```python
from build123d import *

# Parameters (mm, degrees)
SKETCH2_R           = 7.9375
BOSS_EXTRUDE1_DEPTH = 15.875
FILLET1_R           = 12.7
SKETCH3_R           = 22.225
CUT_EXTRUDE1_DEPTH  = 3.175
SKETCH4_R           = 4.7625
CUT_EXTRUDE2_DEPTH  = 6.35
SKETCH5_R           = 3.175
CUT_EXTRUDE3_DEPTH  = 115.871833471
SKETCH6_R           = 1.5875
CUT_EXTRUDE4_DEPTH  = 116.178567885
SKETCH7_W           = 66.04
SKETCH7_H           = 12.7
CUT_EXTRUDE5_DEPTH  = 116.571744492
FILLET2_R           = 3.175


with BuildPart() as part:
    # Sketch2 → Boss-Extrude1 (new body)
    # profile 1 of 5: a face of its own
    with BuildSketch(Plane(origin=(0, 0, 0), x_dir=(1, 0, 0), z_dir=(0, 1, 0))):
        with BuildLine():
            Line((-107.95, 0), (-107.95, -25.4))
            Line((-107.95, -25.4), (-21.997045256, -25.4))
            ThreePointArc((-21.997045256, -25.4), (-25.4, -12.7), (-21.997045256, 0))
            Line((-21.997045256, 0), (-107.95, 0))
        make_face()
    # profile 2 of 5: a face of its own
    with BuildSketch(Plane(origin=(0, 0, 0), x_dir=(1, 0, 0), z_dir=(0, 1, 0))):
        with BuildLine():
            ThreePointArc((-21.997045256, 0), (-25.4, -12.7), (-21.997045256, -25.4))
            Line((-21.997045256, -25.4), (-21.997045256, 0))
        make_face()
    # profile 3 of 5: a face of its own
    with BuildSketch(Plane(origin=(0, 0, 0), x_dir=(1, 0, 0), z_dir=(0, 1, 0))):
        with BuildLine():
            Line((-21.997045256, 0), (-21.997045256, -25.4))
            ThreePointArc((-21.997045256, -25.4), (0, -38.1), (21.997045256, -25.4))
            Line((21.997045256, -25.4), (21.997045256, 0))
            ThreePointArc((21.997045256, 0), (0, 12.7), (-21.997045256, 0))
        make_face()
        with Locations(Location((0, -12.7, 0), (0, 0, 270))):
            Circle(SKETCH2_R, mode=Mode.SUBTRACT)
    # profile 4 of 5: a face of its own
    with BuildSketch(Plane(origin=(0, 0, 0), x_dir=(1, 0, 0), z_dir=(0, 1, 0))):
        with BuildLine():
            Line((21.997045256, 0), (21.997045256, -25.4))
            ThreePointArc((21.997045256, -25.4), (24.534515988, -19.274003746), (25.4, -12.7))
            ThreePointArc((25.4, -12.7), (24.534515988, -6.125996254), (21.997045256, 0))
        make_face()
    # profile 5 of 5: a face of its own
    with BuildSketch(Plane(origin=(0, 0, 0), x_dir=(1, 0, 0), z_dir=(0, 1, 0))):
        with BuildLine():
            ThreePointArc((25.4, -12.7), (24.534515988, -19.274003746), (21.997045256, -25.4))
            Line((21.997045256, -25.4), (107.95, -25.4))
            Line((107.95, -25.4), (107.95, 0))
            Line((107.95, 0), (21.997045256, 0))
            ThreePointArc((21.997045256, 0), (24.534515988, -6.125996254), (25.4, -12.7))
        make_face()
    extrude(amount=BOSS_EXTRUDE1_DEPTH)

    # Fillet1
    fillet1_edges = [part.edges().sort_by_distance(p)[0] for p in [
        (-21.997045256, 7.9375, 0),
        (21.997045256, 7.9375, 0),
        (21.997045256, 7.9375, 25.4),
        (-21.997045256, 7.9375, 25.4),
    ]]
    fillet(fillet1_edges, radius=FILLET1_R)

    # Sketch3 → Cut-Extrude1 (cut)
    with BuildSketch(Plane.XZ):
        with Locations(Location((0, 12.7, 0), (0, 0, 270))):
            Circle(SKETCH3_R)
    extrude(amount=-CUT_EXTRUDE1_DEPTH, mode=Mode.SUBTRACT)

    # Sketch4 → Cut-Extrude2 (cut)
    with BuildSketch(Plane(origin=(0, 15.875, 0), x_dir=(1, 0, 0), z_dir=(0, 1, 0))):
        with Locations(Location((-101.6, -12.7, 0), (0, 0, 270))):
            Circle(SKETCH4_R)
        with Locations(Location((101.6, -12.7, 0), (0, 0, 270))):
            Circle(SKETCH4_R)
    extrude(amount=-CUT_EXTRUDE2_DEPTH, mode=Mode.SUBTRACT)

    # Sketch5 → Cut-Extrude3 (cut, through all)
    with BuildSketch(Plane(origin=(0, 9.525, 0), x_dir=(1, 0, 0), z_dir=(0, 1, 0))):
        with Locations(Location((-101.6, -12.7, 0), (0, 0, 270))):
            Circle(SKETCH5_R)
        with Locations(Location((101.6, -12.7, 0), (0, 0, 270))):
            Circle(SKETCH5_R)
    extrude(amount=-CUT_EXTRUDE3_DEPTH, mode=Mode.SUBTRACT)

    # Sketch6 → Cut-Extrude4 (cut, through all)
    with BuildSketch(Plane.XZ.offset(-3.175)):
        with Locations(Location((0, 29.21, 0), (0, 0, 270))):
            Circle(SKETCH6_R)
        with Locations(Location((14.298079416, 4.445, 0), (0, 0, 270))):
            Circle(SKETCH6_R)
        with Locations(Location((-14.298079416, 4.445, 0), (0, 0, 270))):
            Circle(SKETCH6_R)
    extrude(amount=-CUT_EXTRUDE4_DEPTH, mode=Mode.SUBTRACT)

    # Sketch7 → Cut-Extrude5 (cut, through all)
    with BuildSketch(Plane(origin=(0, 15.875, 0), x_dir=(1, 0, 0), z_dir=(0, 1, 0))):
        with Locations((-58.42, -12.7)):
            Rectangle(SKETCH7_W, SKETCH7_H)
        with Locations((58.42, -12.7)):
            Rectangle(SKETCH7_W, SKETCH7_H)
    extrude(amount=-CUT_EXTRUDE5_DEPTH, mode=Mode.SUBTRACT)

    # Fillet2
    fillet2_edges = [part.edges().sort_by_distance(p)[0] for p in [
        (-91.44, 7.9375, 19.05),
        (-91.44, 7.9375, 6.35),
        (-25.4, 7.9375, 6.35),
        (-25.4, 7.9375, 19.05),
        (25.4, 7.9375, 19.05),
        (25.4, 7.9375, 6.35),
        (91.44, 7.9375, 6.35),
        (91.44, 7.9375, 19.05),
    ]]
    fillet(fillet2_edges, radius=FILLET2_R)


solid = part.part
```
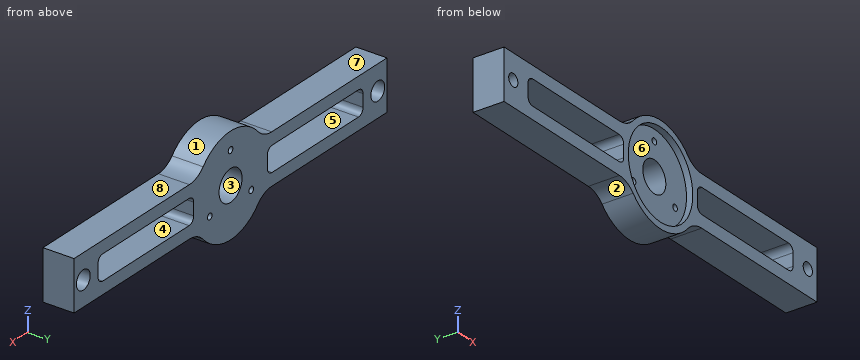
Build history of the part. All positions in model axes, mm. Face numbers are marked on the shaded views. A direction names the side the tool comes from. Round coordinates to 2 decimals unless told otherwise and drop trailing zeros. Loops run counter-clockwise (first coordinate to the right, second up) from the corner with the lowest first, then second, coordinate; pieces in that order, holes last. Notation, with made-up numbers: M 3,81.5 L 38,81.5 A8 cw 38,88.5 Z; hole C 47.5,12.25 d7. An arc over 180 degrees is marked long. Answer as CSV lines item,"result".
1. Flat gauge pins, fed straight in: P1, Ø8, axis at x = -2.5, z = 27.5, coming from the -Y side (3 decimals); P2, Ø1, axis at x = -9, y = 12, coming from the -Z side; P3, Ø5, axis at x = -65.5, y = 4, coming from the -Z side. Where does each tip first touch, or does it go through?
Resolved:
P1,"stops at y = 3.175"
P2,"stops at z = -11.24"
P3,"stops at z = 0"
2. Two-plate mould, pull along X, no slides. Class the marked faces 1, 2, 3 and 4: released by +X, released by -X, zero draft, split by the parting line, or undercut.
Resolved:
face 1,"split by the parting line"
face 2,"released by -X"
face 3,"undercut"
face 4,"undercut"
3. 3-axis set-ups, long thin cutter, end or side, ignore diameter. For the marked faces 5, 6, 7 and 8: which of +Z, -Z, +X, -X, +Y, -Y reach the whole face in a straight line?
Resolved:
face 5,"+Y, -Y"
face 6,"-Y"
face 7,"+Z, -X, +Y, -Y"
face 8,"+Z, +X, +Y, -Y"
4. Wall check: probe 1 along X at (y, z) = (11.25, 12.7); probe 2 along X at (y, z) = (11, 4.5); probe 3 along Z at (x, y) = (-85, 4.25). Give the ranges that are in metal, low to high. Write a range as [from, to].
Resolved:
probe 1,"x = [-107.95, -106.36], [-96.84, -91.44], [-25.4, -7.94], [7.94, 25.4], [91.44, 96.84], [106.36, 107.95]"
probe 2,"x = [-107.95, -15.88], [-12.71, 12.71], [15.88, 107.95]"
probe 3,"z = [0, 6.35], [19.05, 25.4]"
5. Cut at A-A on x = 101.6. Write the cut outline in (y, z) (1 decimal), then the cut area to 3 significant figures.
Resolved:
outline,"M 0,0 L 15.9,0 L 15.9,7.9 L 9.5,7.9 L 9.5,9.5 L 0,9.5 Z; M 0,15.9 L 9.5,15.9 L 9.5,17.5 L 15.9,17.5 L 15.9,25.4 L 0,25.4 Z"
area,"282 mm²"
6. Cut at D-D on z = 22.5. Write the cut outline in (x, y) (3 decimals), then the cut area to 3 significant figures.
Resolved:
outline,"M -107.95,0 L -19.948,0 L -19.948,3.175 L 19.948,3.175 L 19.948,0 L 107.95,0 L 107.95,15.875 L -107.95,15.875 Z"
area,"3,300 mm²"
7. Cut at B-B on z = 12.7. Count the separate pieces of the cut face and the enclosed holes in it, then the cut area to 3 significant figures.
Resolved:
separate pieces,"6"
enclosed holes,"0"
area,"746 mm²"
